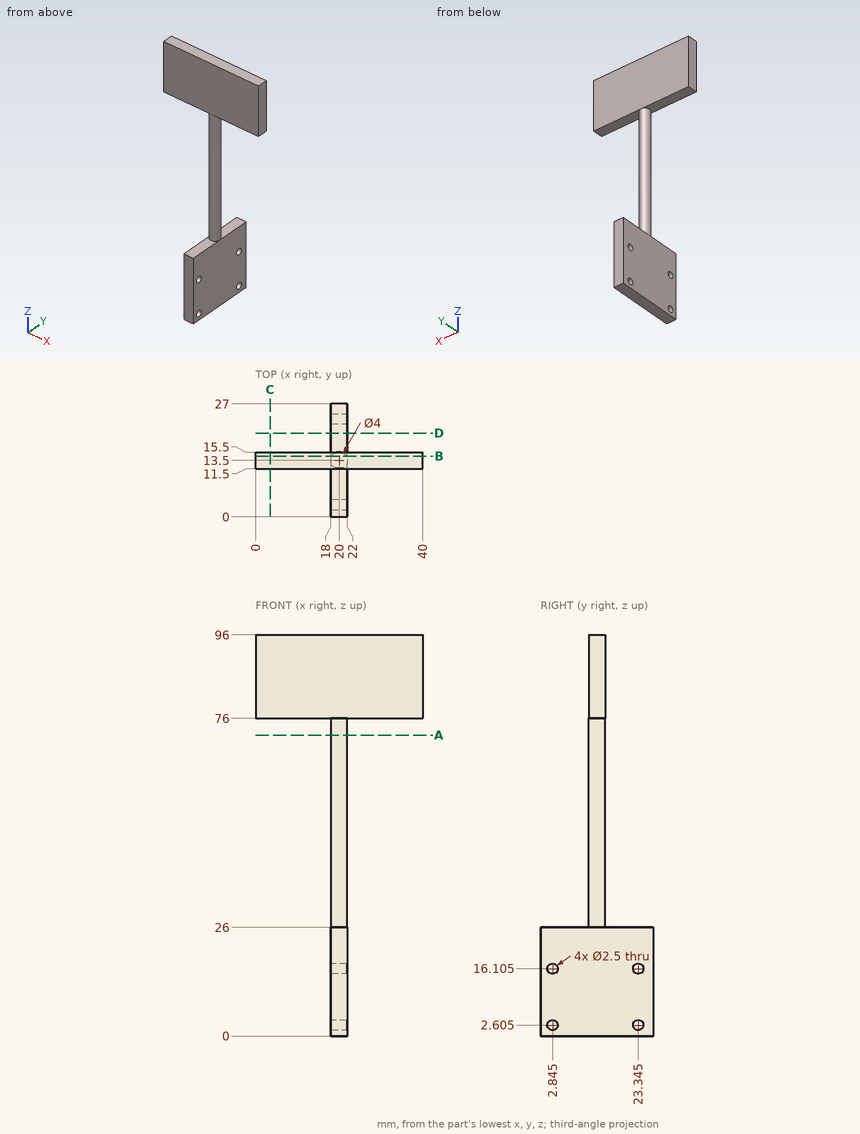
Study the drawing (mm; zero at the part's minimum x, y, z) and answer. Give positions to 0.01 mm unless a question says otherwise; leave off trailing zeros. Loops run counter-clockwise (first coordinate to the right, second up) from the corner with the lowest first, then second, coordinate; pieces in that order, holes last. Notation, with made-up numbers: (78.25, 11) - (114.25, 11) arc R19 cw to (114.25, 21) - close; hole circle Ø9 at (-39, 1.5). An arc over 180 degrees is marked (long way). Answer in a Markdown table with one row per item. Add a question column.
Q1. Consider line 1 along Z through (x, y) = (14, 12.25); line 2 along Y through (x, z) = (30, 83); line 3 along X through (y, z) = (21, 4.5). Determine where each line is inside the solid, lowest interval first.
Q2. The part is cut by section C-C (x = 3.5). Determine the outline of the cut face in (y, z), and give its area (3 significant figures).
Q3. The part is cut by section D-D (y = 20). Determine the outline of the cut face in (x, z).
Q4. Each of these flat-tipped pins is pushed along its axis until it touches: P1, Ø2, axis at x = 19.5, y = 20.5, coming from the +Z side; P2, Ø6, axis at x = 22, z = 87.5, coming from the -Y side; P3, Ø3, axis at y = 23.35, z = 16.1, coming from the +X side; P4, Ø8, axis at x = 24, z = 13.5, coming from the -Y side. Where does it stop, or does it pass through?
Q5. The part is cut by section A-A (z = 72). Determine the outline of the cut face in (x, y).
Q6. The part is cut by section B-B (y = 14.5). Determine the outline of the cut face in (x, z).
Solution:
| question | item | result |
|---|---|---|
| 1 | line 1 | z = 76 to 96 |
| 1 | line 2 | y = 11.5 to 15.5 |
| 1 | line 3 | x = 18 to 22 |
| 2 | outline | (11.5, 76) - (15.5, 76) - (15.5, 96) - (11.5, 96) - close |
| 2 | area | 80.0 mm² |
| 3 | outline | (18, 0) - (22, 0) - (22, 26) - (18, 26) - close |
| 4 | P1 | stops at z = 26 |
| 4 | P2 | stops at y = 11.5 |
| 4 | P3 | stops at x = 22 |
| 4 | P4 | stops at y = 0 |
| 5 | outline | circle Ø4 at (20, 13.5) |
| 6 | outline | (0, 76) - (18.27, 76) - (18.27, 26) - (18, 26) - (18, 0) - (22, 0) - (22, 26) - (21.73, 26) - (21.73, 76) - (40, 76) - (40, 96) - (0, 96) - close |
